Work out the finished part from the listing and answer in its coordinate system (mm). A direction names the side the tool comes from. Give positions to 0.01 mm unless a question says otherwise; leave off trailing zeros. Loops run counter-clockwise (first coordinate to the right, second up) from the corner with the lowest first, then second, coordinate; pieces in that order, holes last. Notation, with made-up numbers: (85.25, -11.5) - (111.25, -11.5) arc R22 cw to (111.25, 9.5) - close; hole circle Ø1 at (28, -8.75). An arc over 180 degrees is marked (long way). One line per question, with ' | ' between items. Start each with the question number.
1. For a pull along X with two mould halves and no side action, classify faces 3 (the face through (53.897, -170.202, 2.348)), 4 (the face through (81.93, -153.32, 2.35)) as released by +X, released by -X, zero draft, split by the parting line, or undercut.
2. This flat-tipped pin is pushed along its axis until it touches: pin 1 (5 mm diameter, centred on x = -6.35, y = -184.15, fed in from +Z). Where does it stop, or does it pass through?
3. Section A-A (y = -215.9) is taken. Determine the outline of the cut face in (x, z), plus the area to 3 significant figures.
4. Section D-D (z = 2.55) is taken. Give the number of separate pieces and of enclosed holes in the cut face, plus the area to 3 significant figures.
5. Section B-B (x = 12.7) is taken. Determine the outline of the cut face in (y, z), plus the area to 3 significant figures.
6. Which of the six approach directions +Z, -Z, +X, -X, +Y, -Y give full straight-line access (tool end or side, diameter ignored) to faces 1 (the face through (121.57, -164.48, 2.35)), 2 (the face through (19.16, -43.3, 2.41))?
7. Find the intervals of material crossed by line 1 (Y direction, x = 107, z = 0.75); line 2 (Y direction, x = -65, z = 3.35); line 3 (Y direction, x = -49, z = 0.8), in increasing order.
8. Section C-C (y = 55.5) is taken. Determine the outline of the cut face in (x, z).
from build123d import *

# Parameters (mm, degrees)
SKETCH1_R           = 3.2639
SKETCH1_R_2         = 14.2875
SKETCH1_R_3         = 2.4892
SKETCH1_R_4         = 12.7
SKETCH1_R_5         = 19.685
BOSS_EXTRUDE1_DEPTH = 4.7625
CUT_EXTRUDE1_DEPTH  = 262.552368382


with BuildPart() as part:
    # Sketch1 → Boss-Extrude1 (new body)
    with BuildSketch(Plane.XY):
        with BuildLine():
            Line((76.2, 0), (76.2, 25.4))
            Line((76.2, 25.4), (50.8, 76.2))
            Line((50.8, 76.2), (12.7, 76.2))
            Line((12.7, 76.2), (-76.2, 76.2))
            Line((-76.2, 76.2), (-76.2, 0))
            Line((-76.2, 0), (-76.2, -228.6))
            Line((-76.2, -228.6), (0, -228.6))
            Line((0, -228.6), (76.2, -228.6))
            Line((76.2, -228.6), (76.2, -222.25))
            ThreePointArc((76.2, -222.25), (79.919743879, -213.269743879), (88.9, -209.55))
            Line((88.9, -209.55), (107.95, -209.55))
            ThreePointArc((107.95, -209.55), (121.420384182, -203.970384182), (127, -190.5))
            Line((127, -190.5), (127, -177.8))
            ThreePointArc((127, -177.8), (121.420384182, -164.329615818), (107.95, -158.75))
            Line((107.95, -158.75), (95.25, -158.75))
            ThreePointArc((95.25, -158.75), (81.779615818, -153.170384182), (76.2, -139.7))
            Line((76.2, -139.7), (76.2, 0))
        make_face()
        with Locations(Location((-38.1, 12.7, 0), (0, 0, 180))):
            Circle(SKETCH1_R, mode=Mode.SUBTRACT)
        with Locations(Location((-12.7, 12.7, 0), (0, 0, 180))):
            Circle(SKETCH1_R, mode=Mode.SUBTRACT)
        with Locations(Location((-63.5, 12.7, 0), (0, 0, 180))):
            Circle(SKETCH1_R, mode=Mode.SUBTRACT)
        with Locations(Location((12.7, 12.7, 0), (0, 0, 180))):
            Circle(SKETCH1_R, mode=Mode.SUBTRACT)
        with Locations(Location((38.1, 12.7, 0), (0, 0, 180))):
            Circle(SKETCH1_R, mode=Mode.SUBTRACT)
        with Locations(Location((38.1, 50.8, 0), (0, 0, 180))):
            Circle(SKETCH1_R_2, mode=Mode.SUBTRACT)
        with Locations(Location((-22.679487758, 32.839487758, 0), (0, 0, 180))):
            Circle(SKETCH1_R_3, mode=Mode.SUBTRACT)
        with Locations(Location((-58.600512242, 32.839487758, 0), (0, 0, 180))):
            Circle(SKETCH1_R_3, mode=Mode.SUBTRACT)
        with Locations(Location((-58.600512242, 68.760512242, 0), (0, 0, 180))):
            Circle(SKETCH1_R_3, mode=Mode.SUBTRACT)
        with Locations(Location((-22.679487758, 68.760512242, 0), (0, 0, 180))):
            Circle(SKETCH1_R_3, mode=Mode.SUBTRACT)
        with Locations(Location((63.5, 12.7, 0), (0, 0, 180))):
            Circle(SKETCH1_R, mode=Mode.SUBTRACT)
        with Locations(Location((-40.64, 50.8, 0), (0, 0, 180))):
            Circle(SKETCH1_R_4, mode=Mode.SUBTRACT)
        with Locations(Location((50.8, -184.15, 0), (0, 0, 180))):
            Circle(SKETCH1_R_2, mode=Mode.SUBTRACT)
        with Locations(Location((63.5, -215.9, 0), (0, 0, 180))):
            Circle(SKETCH1_R, mode=Mode.SUBTRACT)
        with Locations(Location((38.1, -215.9, 0), (0, 0, 180))):
            Circle(SKETCH1_R, mode=Mode.SUBTRACT)
        with Locations(Location((12.7, -215.9, 0), (0, 0, 180))):
            Circle(SKETCH1_R, mode=Mode.SUBTRACT)
        with Locations(Location((50.8, -165.1, 0), (0, 0, 180))):
            Circle(SKETCH1_R_3, mode=Mode.SUBTRACT)
        with Locations(Location((38.1, 69.85, 0), (0, 0, 180))):
            Circle(SKETCH1_R_3, mode=Mode.SUBTRACT)
        with Locations(Location((-6.35, -184.15, 0), (0, 0, 180))):
            Circle(SKETCH1_R, mode=Mode.SUBTRACT)
        with Locations(Location((107.95, -184.15, 0), (0, 0, 180))):
            Circle(SKETCH1_R_2, mode=Mode.SUBTRACT)
        with Locations(Location((107.95, -165.1, 0), (0, 0, 180))):
            Circle(SKETCH1_R_3, mode=Mode.SUBTRACT)
        with Locations(Location((-57.15, -101.6, 0), (0, 0, 180))):
            Circle(SKETCH1_R, mode=Mode.SUBTRACT)
        with Locations(Location((-31.75, -101.6, 0), (0, 0, 180))):
            Circle(SKETCH1_R, mode=Mode.SUBTRACT)
        with Locations(Location((-6.35, -101.6, 0), (0, 0, 180))):
            Circle(SKETCH1_R, mode=Mode.SUBTRACT)
        with Locations(Location((-46.99, -177.8, 0), (0, 0, 180))):
            Circle(SKETCH1_R_5, mode=Mode.SUBTRACT)
        with Locations(Location((-29.029487758, -195.760512242, 0), (0, 0, 180))):
            Circle(SKETCH1_R_3, mode=Mode.SUBTRACT)
        with Locations(Location((-64.950512242, -195.760512242, 0), (0, 0, 180))):
            Circle(SKETCH1_R_3, mode=Mode.SUBTRACT)
        with Locations(Location((-64.950512242, -159.839487758, 0), (0, 0, 180))):
            Circle(SKETCH1_R_3, mode=Mode.SUBTRACT)
        with Locations(Location((-29.029487758, -159.839487758, 0), (0, 0, 180))):
            Circle(SKETCH1_R_3, mode=Mode.SUBTRACT)
        with Locations(Location((-12.7, -215.9, 0), (0, 0, 180))):
            Circle(SKETCH1_R, mode=Mode.SUBTRACT)
        with Locations(Location((-38.1, -215.9, 0), (0, 0, 180))):
            Circle(SKETCH1_R, mode=Mode.SUBTRACT)
        with Locations(Location((-63.5, -215.9, 0), (0, 0, 180))):
            Circle(SKETCH1_R, mode=Mode.SUBTRACT)
    extrude(amount=BOSS_EXTRUDE1_DEPTH)

    # Sketch2 → Cut-Extrude1 (cut, through all)
    with BuildSketch(Plane.XY.offset(4.7625)):
        with BuildLine():
            Line((-12.83077716, -203.2), (19.59926353, -203.2))
            ThreePointArc((19.59926353, -203.2), (25.066064138, -200.300984091), (25.733245747, -194.149149338))
            ThreePointArc((25.733245747, -194.149149338), (25.724761885, -194.127854967), (25.716296113, -194.106553398))
            ThreePointArc((25.716296113, -194.106553398), (23.61470625, -191.486839822), (20.404452937, -190.5))
            Line((20.404452937, -190.5), (-5.477828576, -190.5))
            ThreePointArc((-5.477828576, -190.5), (-6.340017557, -190.434588937), (-7.182470162, -190.239853074))
            Line((-7.182470162, -190.239853074), (-11.035754343, -189.035701768))
            ThreePointArc((-11.035754343, -189.035701768), (-15.003916575, -189.242917347), (-17.877836539, -191.986971616))
            ThreePointArc((-17.877836539, -191.986971616), (-18.23843644, -192.704221477), (-18.616704156, -193.412312704))
            ThreePointArc((-18.616704156, -193.412312704), (-18.515752398, -199.956635736), (-12.83077716, -203.2))
        make_face()
        with BuildLine():
            ThreePointArc((37.978395534, -9.841685227), (37.923146144, -3.269997693), (32.222510687, 0))
            Line((32.222510687, 0), (-33.771257244, 0))
            ThreePointArc((-33.771257244, 0), (-39.298175647, -2.989309284), (-39.821560284, -9.25100758))
            Line((-39.821560284, -9.25100758), (-10.949286814, -75.244775511))
            ThreePointArc((-10.949286814, -75.244775511), (-5.228977015, -79.193518113), (0.856901073, -75.835453158))
            Line((0.856901073, -75.835453158), (37.978395534, -9.841685227))
        make_face()
        with BuildLine():
            ThreePointArc((6.016650935, -104.490665089), (5.959623011, -107.227804875), (7.017552187, -109.752873636))
            Line((7.017552187, -109.752873636), (38.379242123, -155.053092432))
            ThreePointArc((38.379242123, -155.053092432), (41.372935554, -157.43230385), (45.183411581, -157.753426533))
            ThreePointArc((45.183411581, -157.753426533), (45.338775775, -157.720845904), (45.494328922, -157.689179705))
            ThreePointArc((45.494328922, -157.689179705), (49.304178746, -155.399670709), (50.8, -151.214061327))
            Line((50.8, -151.214061327), (50.8, -38.163092112))
            ThreePointArc((50.8, -38.163092112), (45.869462349, -31.774638484), (38.440115153, -34.925406886))
            Line((38.440115153, -34.925406886), (6.201208406, -92.239018879))
            ThreePointArc((6.201208406, -92.239018879), (5.382749443, -94.851548557), (5.694140298, -97.571515859))
            ThreePointArc((5.694140298, -97.571515859), (6.336226337, -101.008678323), (6.016650935, -104.490665089))
        make_face()
        with BuildLine():
            ThreePointArc((28.069846358, -169.60127938), (29.110563089, -165.921638634), (27.937401289, -162.282059163))
            Line((27.937401289, -162.282059163), (0.51656145, -122.674179395))
            ThreePointArc((0.51656145, -122.674179395), (-5.294652738, -119.840268063), (-10.740254608, -123.325477389))
            Line((-10.740254608, -123.325477389), (-24.081589928, -148.340481115))
            ThreePointArc((-24.081589928, -148.340481115), (-24.806096438, -152.278792436), (-23.12177665, -155.911735128))
            ThreePointArc((-23.12177665, -155.911735128), (-17.777951912, -163.819854383), (-14.971403998, -172.94225))
            ThreePointArc((-14.971403998, -172.94225), (-13.046787702, -176.418613316), (-9.321063527, -177.8))
            Line((-9.321063527, -177.8), (20.404452937, -177.8))
            ThreePointArc((20.404452937, -177.8), (23.61470625, -176.813160178), (25.716296113, -174.193446602))
            ThreePointArc((25.716296113, -174.193446602), (26.783063416, -171.840982437), (28.069846358, -169.60127938))
        make_face()
        with BuildLine():
            ThreePointArc((-42.109724533, -145.78482959), (-38.154424423, -145.159684177), (-35.287472281, -142.364010526))
            Line((-35.287472281, -142.364010526), (-25.499607843, -124.011764706))
            ThreePointArc((-25.499607843, -124.011764706), (-25.663783385, -117.506270031), (-31.326666667, -114.3))
            Line((-31.326666667, -114.3), (-44.196, -114.3))
            ThreePointArc((-44.196, -114.3), (-48.865733183, -116.234266817), (-50.8, -120.904))
            Line((-50.8, -120.904), (-50.8, -138.911239606))
            ThreePointArc((-50.8, -138.911239606), (-49.030157857, -143.410543309), (-44.669250814, -145.49826091))
            ThreePointArc((-44.669250814, -145.49826091), (-43.386637762, -145.61609089), (-42.109724533, -145.78482959))
        make_face()
        with BuildLine():
            ThreePointArc((-28.934992756, -88.9), (-23.408074353, -85.910690716), (-22.884689716, -79.64899242))
            Line((-22.884689716, -79.64899242), (-38.14569696, -44.766690148))
            ThreePointArc((-38.14569696, -44.766690148), (-45.548149164, -40.949603929), (-50.8, -47.413697727))
            Line((-50.8, -47.413697727), (-50.8, -82.296))
            ThreePointArc((-50.8, -82.296), (-48.865733183, -86.965733183), (-44.196, -88.9))
            Line((-44.196, -88.9), (-28.934992756, -88.9))
        make_face()
    extrude(amount=-CUT_EXTRUDE1_DEPTH, mode=Mode.SUBTRACT)


solid = part.part
Conclusion:
1) face 3: undercut | face 4: released by +X
2) pin 1: through
3) outline: (-76.2, 0) - (-66.76, 0) - (-66.76, 4.76) - (-76.2, 4.76) - close; (-60.24, 0) - (-41.36, 0) - (-41.36, 4.76) - (-60.24, 4.76) - close; (-34.84, 0) - (-15.96, 0) - (-15.96, 4.76) - (-34.84, 4.76) - close; (-9.44, 0) - (9.44, 0) - (9.44, 4.76) - (-9.44, 4.76) - close; (15.96, 0) - (34.84, 0) - (34.84, 4.76) - (15.96, 4.76) - close; (41.36, 0) - (60.24, 0) - (60.24, 4.76) - (41.36, 4.76) - close; (66.76, 0) - (77.9, 0) - (77.9, 4.76) - (66.76, 4.76) - close | area: 547 mm²
4) separate pieces: 1 | enclosed holes: 38 | area: 32,300 mm²
5) outline: (-228.6, 0) - (-219.16, 0) - (-219.16, 4.76) - (-228.6, 4.76) - close; (-212.64, 0) - (-203.2, 0) - (-203.2, 4.76) - (-212.64, 4.76) - close; (-190.5, 0) - (-177.8, 0) - (-177.8, 4.76) - (-190.5, 4.76) - close; (-140.27, 0) - (-117.96, 0) - (-117.96, 4.76) - (-140.27, 4.76) - close; (-80.69, 0) - (-54.78, 0) - (-54.78, 4.76) - (-80.69, 4.76) - close; (0, 0) - (9.44, 0) - (9.44, 4.76) - (0, 4.76) - close; (15.96, 0) - (76.2, 0) - (76.2, 4.76) - (15.96, 4.76) - close | area: 712 mm²
6) face 1: +Z, -Z, +X, +Y | face 2: +Z, -Z
7) line 1: -209.55 to -198.41, -169.89 to -167.4, -162.8 to -158.75 | line 2: -228.6 to -218.8, -213 to -198.25, -193.27 to -185.75, -169.85 to -162.33, -157.35 to 9.8, 15.6 to 76.2 | line 3: -228.6 to -197.38, -158.22 to -143.44, -116.37 to -86.83, -42.88 to 41.24, 60.36 to 76.2
8) outline: (-76.2, 0) - (-52.44, 0) - (-52.44, 4.76) - (-76.2, 4.76) - close; (-28.84, 0) - (24.61, 0) - (24.61, 4.76) - (-28.84, 4.76) - close; (51.59, 0) - (61.15, 0) - (61.15, 4.76) - (51.59, 4.76) - close
